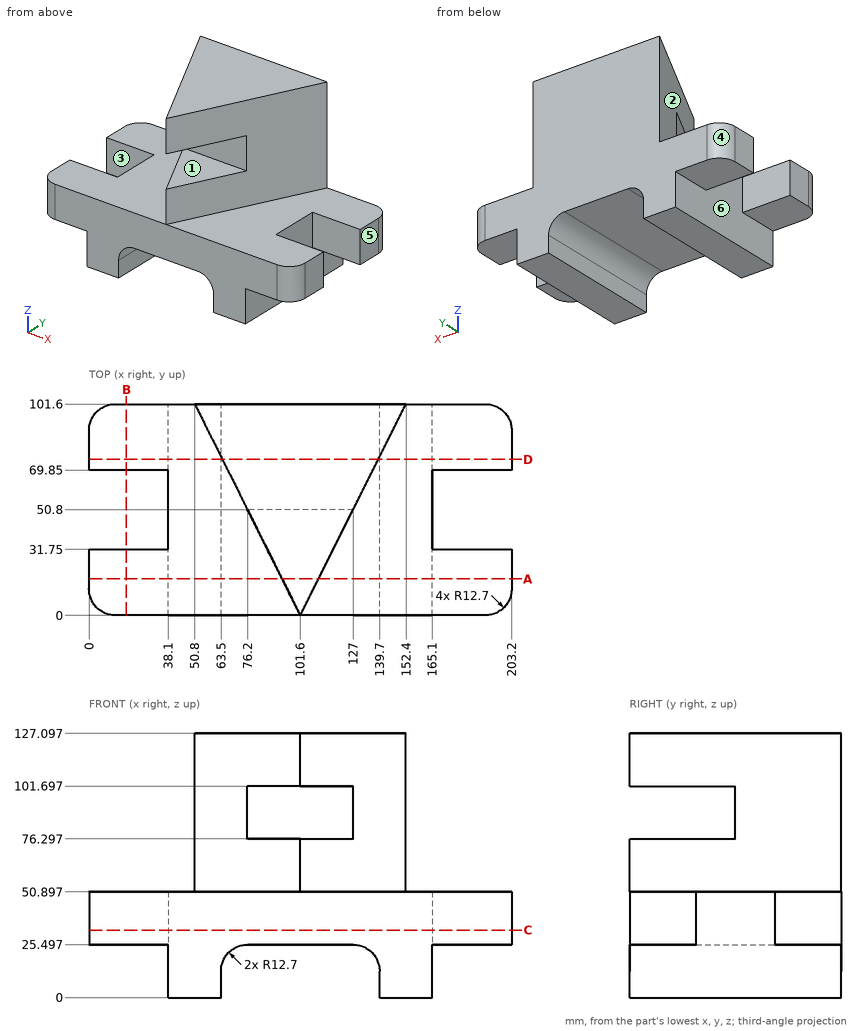
Input: dimensioned drawing with shaded views. Units: mm. Origin: part minimum x, y, z. A direction names the side the tool comes from. Round coordinates to 2 decimals unless told otherwise and drop trailing zeros. Order: outer loops, then holes, each group sorted by start corner. A loop starts at its lowest first (then second) coordinate and runs counter-clockwise, first axis right, second up. Notation, with made-up numbers: (10, 44.5) -> (26, 44.5) arc R8 ccw to (26, 55.5) -> close; hole circle Ø2 at (-6, 35). An arc over 180 degrees is marked (long way). Put each result on its own line as item: value. Start each with the question number.
Q1. Section B-B on x = 18. Return the cut outline in (y, z).
Q2. Pull-direction query (Y, two-part tool) for the marked faces 4, 5 and 6; classes: +Y half, -Y half, draft (parallel to the pull), parting line (faces both ways), or undercut.
Q3. Section A-A on y = 17.5. Return the cut outline in (x, z), and give its area (3 significant figures).
Q4. Section C-C on z = 32.5. Return the cut outline in (x, y), and give its area (3 significant figures).
Q5. Section D-D on y = 75. Return the cut outline in (x, z), and give its area (3 significant figures).
Q6. First-contact query: pin 1 (3 mm diameter, centred on x = 74, y = 68, fed in from -Z); pin 2 (8 mm diameter, centred on y = 50, z = 69.5, fed in from -X); pin 3 (10 mm diameter, centred on x = 94, y = 81.5, fed in from -Z). Flat tips, straight axial feed; report the tip coordinate or a pass-through.
Q7. Reachability of the marked faces 1, 2 and 3 from +Z, -Z, +X, -X, +Y, -Y: full face, straight path, thin tool, end or side. Return the list, or none.
Q8. Line query: probe 1 along X at (y, z) = (79, 6); probe 2 along Z at (x, y) = (121.5, 65); probe 3 along X at (y, z) = (37, 26). Output: solid intervals per line, ascending.
Ans:
1. outline: (0, 25.5) -> (31.75, 25.5) -> (31.75, 50.9) -> (0, 50.9) -> close; (69.85, 25.5) -> (101.6, 25.5) -> (101.6, 50.9) -> (69.85, 50.9) -> close
2. face 4: +Y half
2. face 5: draft
2. face 6: undercut
3. outline: (0, 25.5) -> (38.1, 25.5) -> (38.1, 0) -> (63.5, 0) -> (63.5, 12.8) arc R12.7 cw to (76.2, 25.5) -> (127, 25.5) arc R12.7 cw to (139.7, 12.8) -> (139.7, 0) -> (165.1, 0) -> (165.1, 25.5) -> (203.2, 25.5) -> (203.2, 50.9) -> (110.35, 50.9) -> (110.35, 76.3) -> (92.85, 76.3) -> (92.85, 50.9) -> (0, 50.9) -> close; (92.85, 101.7) -> (110.35, 101.7) -> (110.35, 127.1) -> (92.85, 127.1) -> close
3. area: 7,410 mm2
4. outline: (0, 12.7) arc R12.7 ccw to (12.7, 0) -> (190.5, 0) arc R12.7 ccw to (203.2, 12.7) -> (203.2, 31.75) -> (165.1, 31.75) -> (165.1, 69.85) -> (203.2, 69.85) -> (203.2, 88.9) arc R12.7 ccw to (190.5, 101.6) -> (12.7, 101.6) arc R12.7 ccw to (0, 88.9) -> (0, 69.85) -> (38.1, 69.85) -> (38.1, 31.75) -> (0, 31.75) -> close
4. area: 17,600 mm2
5. outline: (0, 25.5) -> (38.1, 25.5) -> (38.1, 0) -> (63.5, 0) -> (63.5, 12.8) arc R12.7 cw to (76.2, 25.5) -> (127, 25.5) arc R12.7 cw to (139.7, 12.8) -> (139.7, 0) -> (165.1, 0) -> (165.1, 25.5) -> (203.2, 25.5) -> (203.2, 50.9) -> (139.1, 50.9) -> (139.1, 127.1) -> (64.1, 127.1) -> (64.1, 50.9) -> (0, 50.9) -> close
5. area: 12,200 mm2
6. pin 1: stops at z = 24.95
6. pin 2: stops at x = 74.6
6. pin 3: stops at z = 25.5
7. face 1: +X, -X, -Y
7. face 2: +Z, -X, -Y
7. face 3: +Z, -Z, -X
8. probe 1: x = 38.1 to 63.5, 139.7 to 165.1
8. probe 2: z = 25.5 to 127.1
8. probe 3: x = 38.1 to 165.1
